The model under review builds one solid part; all positions refer to its coordinate system, in mm. A direction names the side the tool comes from. Coordinates: 2 decimals unless noted, no trailing zeros. Order: outer loops, then holes, each group sorted by start corner. A loop starts at its lowest first (then second) coordinate and runs counter-clockwise, first axis right, second up. Notation, with made-up numbers: (5.5, 1.5) -> (57.5, 1.5) arc R9 ccw to (57.5, 11.5) -> close; hole circle Ø2 at (5, 23). An arc over 180 degrees is marked (long way). Use one line per item in the form item = value.
Solid Edge part; units mm, degrees
sketch "Sketch1" plane through (0, 0, 0) normal (0, 0, 1) x (1, 0, 0)
  line L0 (7.9496, 35.9141) -> (11.9215, 1.3707)
  line L1 (-7.9496, 35.9141) -> (-11.9215, 1.3707)
  arc A0 (11.9215, 1.3707) -> (-11.9215, 1.3707) centre (0, 0) cw
  arc A1 (-7.9496, 35.9141) -> (7.9496, 35.9141) centre (0, 35) cw
extrude "Protrusion1" add sketch "Sketch1" along normal mid plane 6
sketch "Sketch2" plane through (0, 0, 0) normal (0, 0, 1) x (1, 0, 0)
  circle A0 centre (0, 0) radius 8
extrude "ExtrudedCutout_1" cut sketch "Sketch2" along normal blind 28.5335
sketch "Sketch3" plane through (0, 0, 0) normal (0, 0, 1) x (1, 0, 0)
  circle A0 centre (-5.068, 0) radius 1.75
  circle A1 centre (5.068, 0) radius 1.75
extrude "ExtrudedCutout_2" cut sketch "Sketch3" along normal mid plane 265.7863
sketch "Sketch4" plane through (0, 0, 0) normal (0, 0, 1) x (1, 0, 0)
  circle A0 centre (0, 35) radius 4
extrude "ExtrudedCutout_3" cut sketch "Sketch4" along normal mid plane 190.7262
sketch "Sketch5" plane through (0, 0, 0) normal (0, 0, 1) x (1, 0, 0)
  circle A0 centre (0, 35) radius 8.002
extrude "ExtrudedProtrusion_2" add sketch "Sketch5" along normal blind 5
sketch "Sketch6" plane through (0, 0, 0) normal (0, 0, 1) x (1, 0, 0)
  circle A0 centre (0, 35) radius 4
extrude "ExtrudedCutout_4" cut sketch "Sketch6" along normal mid plane 58.2949
sketch "Sketch7" plane through (0, 0, 0) normal (0, 0, 1) x (1, 0, 0)
  line L0 (-1.9, 8.5724) -> (1.9, 8.5724)
  line L1 (1.9, 8.5724) -> (1.9, -8.5724)
  line L2 (1.9, -8.5724) -> (-1.9, -8.5724)
  line L3 (-1.9, -8.5724) -> (-1.9, 8.5724)
extrude "ExtrudedProtrusion_4" add sketch "Sketch7" along normal blind 2.95
Item 1: Tool access review of faces 1 (the face through (0, 0, 2.95)), 2 (the face through (6.737, 0.526, -1.479)): name each direction out of +Z, -Z, +X, -X, +Y, -Y from which nothing blocks a thin tool from reaching the whole face with its end or side.
Results found:
face_1 = +Z
face_2 = +Z, -Z
Item 2: We need section C-C (y = 0). Write out the cut boundary in (x, z).
Results found:
outline = (-12, -3) -> (-6.82, -3) -> (-6.82, 0) -> (-8, 0) -> (-8, 3) -> (-12, 3) -> close; (-3.32, -3) -> (3.32, -3) -> (3.32, 0) -> (1.9, 0) -> (1.9, 2.95) -> (-1.9, 2.95) -> (-1.9, 0) -> (-3.32, 0) -> close; (6.82, -3) -> (12, -3) -> (12, 3) -> (8, 3) -> (8, 0) -> (6.82, 0) -> close
Item 3: We need section D-D (y = 35). Write out the cut boundary in (x, z), plus the area to 3 significant figures.
Results found:
outline = (-8.05, -3) -> (-4, -3) -> (-4, 5) -> (-8, 5) -> (-8, 3) -> (-8.05, 3) -> close; (4, -3) -> (8.05, -3) -> (8.05, 3) -> (8, 3) -> (8, 5) -> (4, 5) -> close
area = 64.7 mm²
Item 4: We need section B-B (x = 0). Write out the cut boundary in (y, z), plus the area to 3 significant figures.
Results found:
outline = (-12, -3) -> (31, -3) -> (31, 5) -> (27, 5) -> (27, 3) -> (8, 3) -> (8, 2.95) -> (-8, 2.95) -> (-8, 3) -> (-12, 3) -> close; (39, -3) -> (43, -3) -> (43, 5) -> (39, 5) -> close
area = 297 mm²
Item 5: We need section A-A (z = 0.75). Write out the cut boundary in (x, y), plus the area to 3 significant figures.
Results found:
outline = (-11.92, 1.37) arc R12 ccw (long way) to (11.92, 1.37) -> (7.95, 35.91) arc R8 ccw to (-7.95, 35.91) -> close; hole circle Ø8 at (0, 35); hole (-1.9, -7.77) -> (-1.9, 7.77) arc R8 ccw to start; hole (1.9, -7.77) arc R8 ccw to (1.9, 7.77) -> close
area = 840 mm²
Item 6: Draft analysis for pull direction Y (two halves, no side actions). For faces 3 (the face through (7.39, 3.06, 1.48)), 4 (the face through (-1.9, 0, 1)), 5 (the face through (2, 39, 5)), 6 (the face through (-1.735, 42.812, 1.833)), state which applies: released by +Y, released by -Y, zero draft, split by the parting line, or undercut.
Results found:
face_3 = undercut
face_4 = undercut
face_5 = zero draft
face_6 = split by the parting line
Item 7: Clearance check with flat-ended pins moving along their axes: pin 1 (4.5 mm diameter, centred on x = 5.068, y = 0, fed in from -Z); pin 2 (8 mm diameter, centred on x = -4, y = 16.5, fed in from +Z); pin 3 (3 mm diameter, centred on x = 8.5, z = 1, fed in from -Y); pin 4 (1.8 mm diameter, centred on x = -5, y = -2.5, fed in from +Z). State where each tip first meets the part, or that it passes through.
Results found:
pin_1 = -3
pin_2 = 3
pin_3 = -9.75
pin_4 = 0
Item 8: To check wall thickness, follow L1, parallel to X at y = 0, z = 2.15; L2, parallel to X at y = 4.5, z = 2.25; L3, parallel to Y at x = 2.25, z = 1.5. State the ranges of each line that lie inside material, in increasing order. Write a range as from..to.
Results found:
L1 = -12..-8, -1.9..1.9, 8..12
L2 = -11.56..-6.61, -1.9..1.9, 6.61..11.56
L3 = -11.79..-7.68, 7.68..31.69, 38.31..42.68
